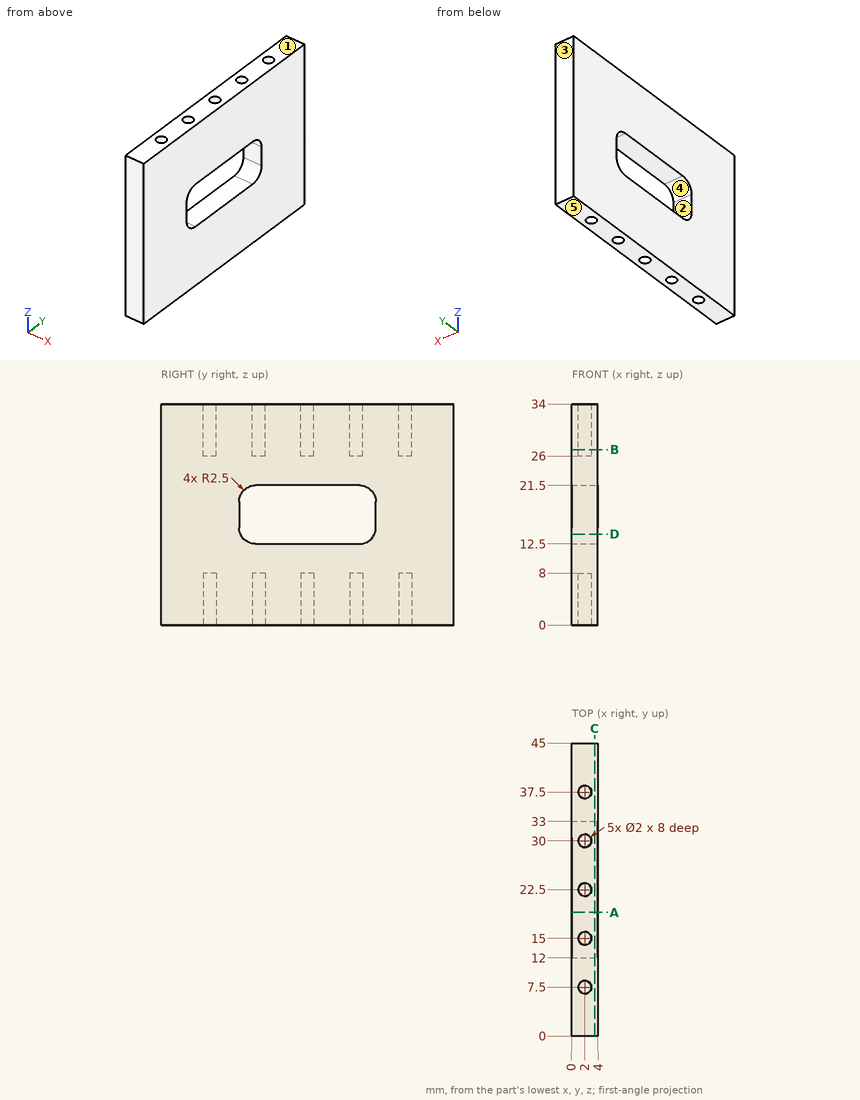
The figure shows three views and two pictorial views of one solid part (mm, origin at its lowest corner). Answer the questions. A direction names the side the tool comes from. Round coordinates to 2 decimals unless told otherwise and drop trailing zeros. Loops run counter-clockwise (first coordinate to the right, second up) from the corner with the lowest first, then second, coordinate; pieces in that order, holes last. Notation, with made-up numbers: M 75.5,-37.5 L 79.5,-37.5 A23 cw 79.5,-28.5 Z; hole C 2.5,-28.5 d8. An arc over 180 degrees is marked long. Write each question's results on one line, items separated by ' | '. Start each with the question number.
1) Find section A-A on y = 19. Write down the section's boundary in (x, z), plus the area to 3 significant figures.
2) Determine the mould class of the marked faces 3, 4 and 5 for opening direction Z: pulls with the +Z half, pulls with the -Z half, needs draft (parallel to the pull), parting line crosses it, or undercut.
3) Which of the six approach directions +Z, -Z, +X, -X, +Y, -Y give full straight-line access (tool end or side, diameter ignored) to the marked faces 1 and 2?
4) Find section C-C on x = 3.5. Write down the section's boundary in (y, z).
5) Find section B-B on z = 27. Write down the section's boundary in (x, y).
6) Each of these flat-tipped pins is pushed along its axis until it touches: pin 1 (5 mm diameter, centred on y = 24.5, z = 7.5, fed in from -X); pin 2 (1 mm diameter, centred on x = 2, y = 30, fed in from -Z); pin 3 (1.6 mm diameter, centred on x = 2, y = 7.5, fed in from +Z). Where does it stop, or does it pass through?
7) Find section D-D on z = 14. Write down the section's boundary in (x, y).
8) Straight lines are drawn through the part: probe 1 along Y at (x, z) = (2, 29.25); probe 2 along Z at (x, y) = (2.8, 17.5); probe 3 along Y at (x, z) = (1.55, 18). For each, find the intervals that lie inside material, in ascending order.
Final values:
1) outline: M 0,0 L 4,0 L 4,12.5 L 0,12.5 Z; M 0,21.5 L 4,21.5 L 4,34 L 0,34 Z | area: 100 mm²
2) face 3: needs draft | face 4: undercut | face 5: pulls with the -Z half
3) face 1: +Z, +X, -X, +Y, -Y | face 2: +X, -X
4) outline: M 0,0 L 45,0 L 45,34 L 0,34 Z; hole M 12,15 A2.5 ccw 14.5,12.5 L 30.5,12.5 A2.5 ccw 33,15 L 33,19 A2.5 ccw 30.5,21.5 L 14.5,21.5 A2.5 ccw 12,19 Z
5) outline: M 0,0 L 4,0 L 4,45 L 0,45 Z; hole C 2,7.5 d2; hole C 2,15 d2; hole C 2,22.5 d2; hole C 2,30 d2; hole C 2,37.5 d2
6) pin 1: x = 0 | pin 2: z = 8 | pin 3: z = 26
7) outline: M 0,0 L 4,0 L 4,12.21 L 0,12.21 Z; M 0,32.79 L 4,32.79 L 4,45 L 0,45 Z
8) probe 1: 0 to 6.5, 8.5 to 14, 16 to 21.5, 23.5 to 29, 31 to 36.5, 38.5 to 45 | probe 2: 0 to 12.5, 21.5 to 34 | probe 3: 0 to 12, 33 to 45
